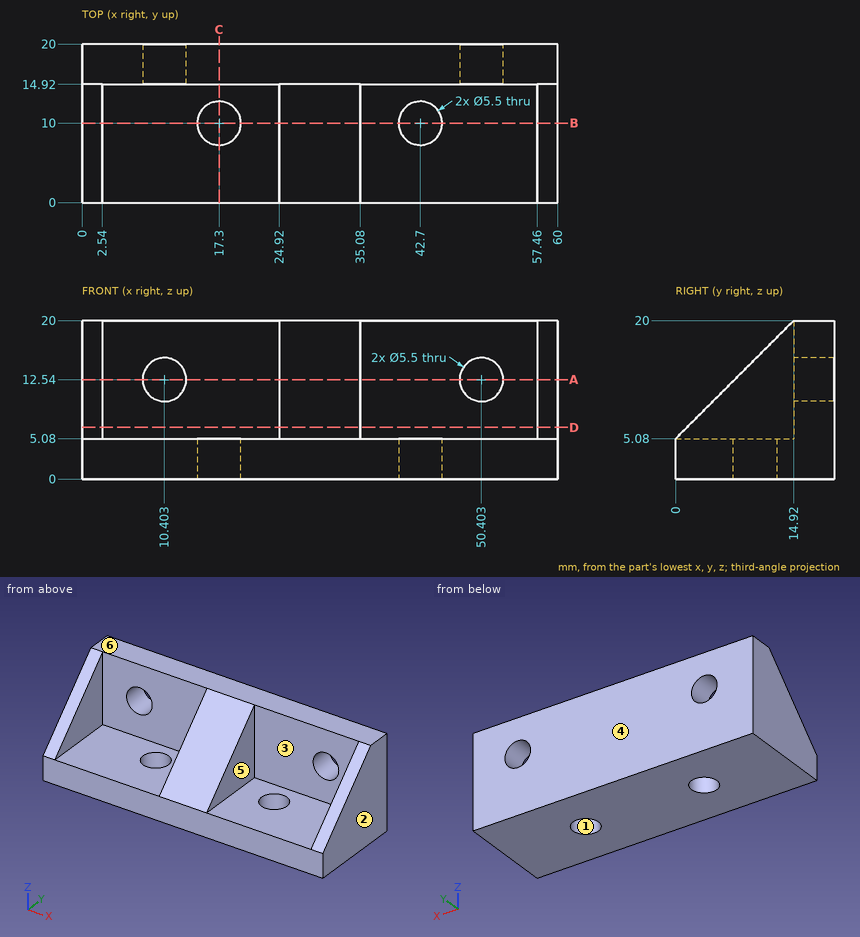
For this review, use the dimensioned drawing (mm, ordinates from the lowest corner) and the shaded views. A direction names the side the tool comes from. Give positions to 0.01 mm unless a question says otherwise; leave off trailing zeros. Order: outer loops, then holes, each group sorted by start corner. A loop starts at its lowest first (then second) coordinate and runs counter-clockwise, first axis right, second up. Notation, with made-up numbers: M -25,-24 L 26,-24 A13 cw 26,-20 Z; hole C 22.25,-37.75 d8. An arc over 180 degrees is marked long. Use one line per item in the form item = value. Start each with the question number.
Item 1: We need section B-B on y = 10. Give the boundary of the cut face in (x, z).
Item 2: We need section D-D on z = 6.5. Give the boundary of the cut face in (x, y).
Item 3: For the marked faces 5 and 6, list the 3-axis set-ups (+Z, -Z, +X, -X, +Y, -Y) from which the entire face can be reached by the end or side of a thin tool; tool diameter is ignored.
Item 4: The part is to be moulded in two halves that separate along Y. For the marked faces 1, 2, 3 and 4, say which applies: pulls with the +Y half, pulls with the -Y half, needs draft (parallel to the pull), parting line crosses it, or undercut.
Item 5: We need section A-A on z = 12.54. Give the boundary of the cut face in (x, y).
Item 6: We need section C-C on x = 17.3. Give the boundary of the cut face in (y, z).
Item 7: To check wall thickness, follow line 1 along X through (y, z) = (14.25, 8); line 2 along X through (y, z) = (9.5, 3.75) (1 decimal); line 3 along Z through (x, y) = (51, 12). State the ranges of each line that lie inside material, in increasing order. Write a range as from..to.
Item 8: Insertion check: pin 1 Ø8 at (x, z) = (23, 8.5) entering from -Y; pin 2 Ø7.5 at (x, y) = (46.5, 10) entering from +Z; pin 3 Ø10 at (y, z) = (3.5, 17.5) entering from +X; pin 4 Ø12 at (x, z) = (43, 13.5) entering from -Y. Each pin has a flat end and moves straight along its axis. Give the tip position at first contact, or say it passes through.
Completed:
q1.outline = M 0,0 L 14.55,0 L 14.55,5.08 L 2.54,5.08 L 2.54,15.08 L 0,15.08 Z; M 20.05,0 L 39.95,0 L 39.95,5.08 L 35.08,5.08 L 35.08,15.08 L 24.92,15.08 L 24.92,5.08 L 20.05,5.08 Z; M 45.45,0 L 60,0 L 60,15.08 L 57.46,15.08 L 57.46,5.08 L 45.45,5.08 Z
q2.outline = M 0,1.42 L 2.54,1.42 L 2.54,14.92 L 24.92,14.92 L 24.92,1.42 L 35.08,1.42 L 35.08,14.92 L 57.46,14.92 L 57.46,1.42 L 60,1.42 L 60,20 L 0,20 Z
q3.face_5 = +Z, -Y
q3.face_6 = +Z, +X, -X, +Y, -Y
q4.face_1 = undercut
q4.face_2 = needs draft
q4.face_3 = pulls with the -Y half
q4.face_4 = pulls with the +Y half
q5.outline = M 0,7.46 L 2.54,7.46 L 2.54,14.92 L 7.65,14.92 L 7.65,20 L 0,20 Z; M 13.15,14.92 L 24.92,14.92 L 24.92,7.46 L 35.08,7.46 L 35.08,14.92 L 47.65,14.92 L 47.65,20 L 13.15,20 Z; M 53.15,14.92 L 57.46,14.92 L 57.46,7.46 L 60,7.46 L 60,20 L 53.15,20 Z
q6.outline = M 0,0 L 7.25,0 L 7.25,5.08 L 0,5.08 Z; M 12.75,0 L 20,0 L 20,20 L 14.92,20 L 14.92,5.08 L 12.75,5.08 Z
q7.line_1 = 0..2.54, 24.92..35.08, 57.46..60
q7.line_2 = 0..14.6, 20..40, 45.4..60
q7.line_3 = 0..5.08
q8.pin_1 = 0
q8.pin_2 = 5.08
q8.pin_3 = through
q8.pin_4 = 14.92
